Check sheet for the drawn part. Datum: minimum x, y, z corner. Units: mm. A direction names the side the tool comes from. Round coordinates to 2 decimals unless told otherwise and drop trailing zeros. Write each loop counter-clockwise with the first axis right and the second up, starting at its lowest first coordinate (ties: lowest second). Pieces come first, ordered by that corner, then holes. Notation, with made-up numbers: M 26.5,21.5 L 47.5,21.5 A8 cw 47.5,27.5 Z; hole C 27,36.25 d3. An arc over 180 degrees is marked long. One line per item, written item: value.
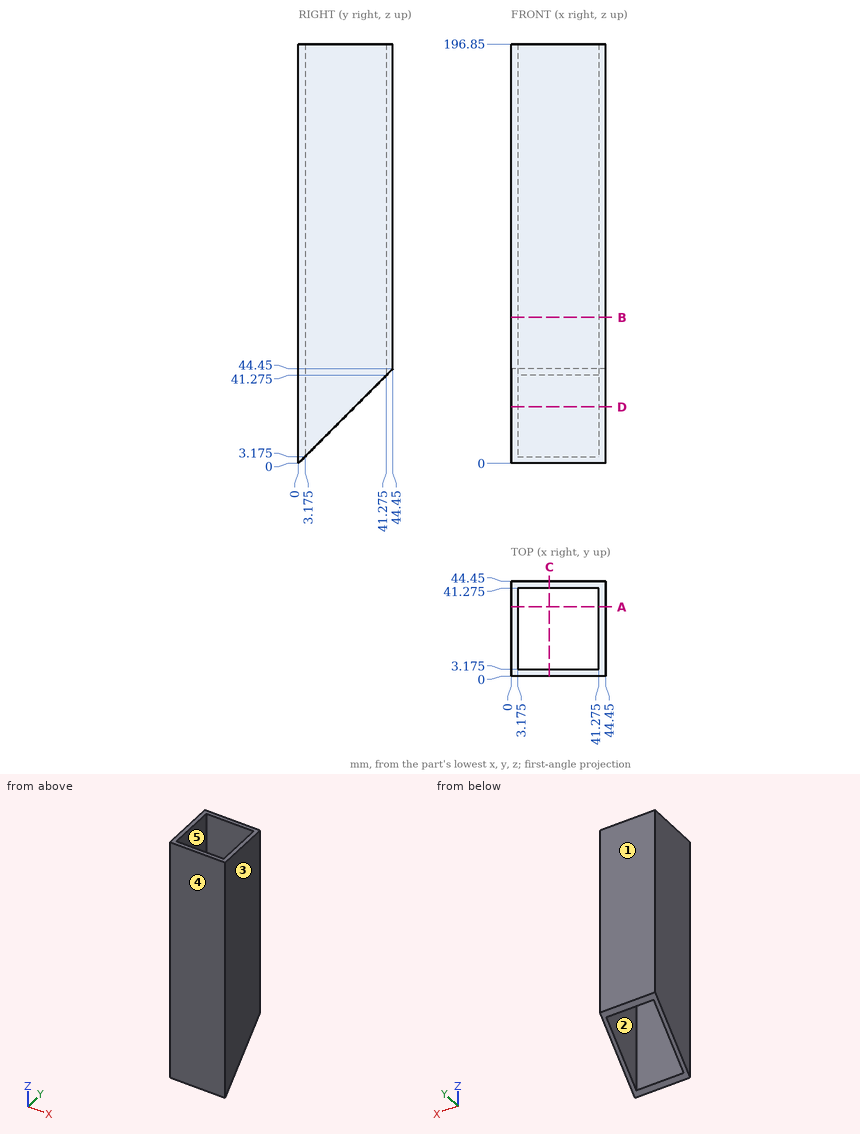
Q1. Access from +Z, -Z, +X, -X, +Y, -Y to the whole of each face (thin tool, end or side, straight path). Record for the marked faces 1 and 2.
Completed:
face 1: +Z, -Z, +X, -X, +Y
face 2: +Z, -Z
Q2. Sectioned sample at B-B on z = 68.5. Enter the section's corners in (x, y) (3 decimals).
Completed:
outline: M 0,0 L 44.45,0 L 44.45,44.45 L 0,44.45 Z; hole M 3.175,3.175 L 41.275,3.175 L 41.275,41.275 L 3.175,41.275 Z
Q3. Draft check along X on the marked faces 3, 4 and 5. Enter one of: pulls with the +X half, pulls with the -X half, needs draft (parallel to the pull), parting line crosses it, or undercut.
Completed:
face 3: pulls with the +X half
face 4: needs draft
face 5: undercut
Q4. Sectioned sample at A-A on y = 32.5. Enter the section's corners in (x, z) (3 decimals), and give its area (3 significant figures).
Completed:
outline: M 0,32.5 L 3.175,32.5 L 3.175,196.85 L 0,196.85 Z; M 41.275,32.5 L 44.45,32.5 L 44.45,196.85 L 41.275,196.85 Z
area: 1,040 mm^2
Q5. Sectioned sample at D-D on z = 26.5. Enter the section's corners in (x, y) (3 decimals), and give its area (3 significant figures).
Completed:
outline: M 0,0 L 44.45,0 L 44.45,26.5 L 41.275,26.5 L 41.275,3.175 L 3.175,3.175 L 3.175,26.5 L 0,26.5 Z
area: 289 mm^2
Q6. Scan lines: line 1 (X direction, y = 35, z = 62.5) (3 decimals); line 2 (Y direction, x = 33, z = 18) (3 decimals). Record each from-to range of solid material in increasing order. Write a range as [from, to].
Completed:
line 1: [0, 3.175], [41.275, 44.45]
line 2: [0, 3.175]
Q7. Sectioned sample at C-C on x = 18. Enter the section's corners in (y, z) (3 decimals), and give its area (3 significant figures).
Completed:
outline: M 0,0 L 3.175,3.175 L 3.175,196.85 L 0,196.85 Z; M 41.275,41.275 L 44.45,44.45 L 44.45,196.85 L 41.275,196.85 Z
area: 1,110 mm^2
